```python
from build123d import *

# Parameters (mm, degrees)
ESQUISSE1_R             = 3
BOSS_EXTRU_1_DEPTH      = 10
ESQUISSE2_R             = 2
BOSS_EXTRU_2_DEPTH      = 8
ESQUISSE6_W             = 50
ESQUISSE6_H             = 0.42
BOSS_EXTRU_4_DEPTH      = 10
ESQUISSE7_W             = 50
ESQUISSE7_H             = 0.81
ENL_V_MAT_EXTRU_3_DEPTH = 10
ESQUISSE8_R             = 2
BOSS_EXTRU_5_DEPTH      = 8.39


with BuildPart() as part:
    # Esquisse1 → Boss.-Extru.1 (new body)
    with BuildSketch(Plane.XY):
        with BuildLine():
            Line((-25, -12.35), (25, -12.35))
            Line((25, -12.35), (25, 12.35))
            ThreePointArc((25, 12.35), (0, 37.35), (-25, 12.35))
            Line((-25, 12.35), (-25, -12.35))
        make_face()
        with Locations((0, 12.35)):
            Circle(ESQUISSE1_R, mode=Mode.SUBTRACT)
    extrude(amount=BOSS_EXTRU_1_DEPTH)

    # Esquisse2 → Boss.-Extru.2 (add)
    with BuildSketch(Plane.XZ.offset(12.35)):
        with Locations(Location((-10.94600496, 5, 0), (0, 0, 90))):
            Circle(ESQUISSE2_R)
        with Locations(Location((10.94600496, 5, 0), (0, 0, 90))):
            Circle(ESQUISSE2_R)
    extrude(amount=BOSS_EXTRU_2_DEPTH)

    # Esquisse6 → Boss.-Extru.4 (add)
    with BuildSketch(Plane.XY.offset(10)):
        with Locations((0, -12.56)):
            Rectangle(ESQUISSE6_W, ESQUISSE6_H)
    extrude(amount=-BOSS_EXTRU_4_DEPTH)

    # Esquisse7 → Enl_v. mat.-Extru.3 (cut)
    with BuildSketch(Plane.XY.offset(10)):
        with Locations((0, -12.365)):
            Rectangle(ESQUISSE7_W, ESQUISSE7_H)
    extrude(amount=-ENL_V_MAT_EXTRU_3_DEPTH, mode=Mode.SUBTRACT)


with BuildPart() as enl_v_mat_extru_3_piece_1:
    # of the separate pieces the step leaves, piece 1, a body of its own (enl_v_mat_extru_3_pieces)
    add(part.part.solids().sort_by_distance((-25, 12.35, 0))[0])



with BuildPart() as enl_v_mat_extru_3_piece_2:
    # of the separate pieces the step leaves, piece 2, a body of its own (enl_v_mat_extru_3_pieces)
    add(part.part.solids().sort_by_distance((-10.94600496, -12.77, 7))[0])


with BuildPart() as enl_v_mat_extru_3_piece_3:
    # of the separate pieces the step leaves, piece 3, a body of its own (enl_v_mat_extru_3_pieces)
    add(part.part.solids().sort_by_distance((10.94600496, -12.77, 7))[0])


with BuildPart() as enl_v_mat_extru_3_piece_1_1:
    add(enl_v_mat_extru_3_piece_1.part)

    add(enl_v_mat_extru_3_piece_2.part)  # Boss.-Extru.5 merges Enl_v. mat.-Extru.3 piece 2

    add(enl_v_mat_extru_3_piece_3.part)  # Boss.-Extru.5 merges Enl_v. mat.-Extru.3 piece 3
    # Esquisse8 → Boss.-Extru.5 (add)
    with BuildSketch(Plane.XZ.offset(11.96)):
        with Locations(Location((-10.94600496, 5, 0), (0, 0, 90))):
            Circle(ESQUISSE8_R)
        with Locations(Location((10.94600496, 5, 0), (0, 0, 90))):
            Circle(ESQUISSE8_R)
    extrude(amount=BOSS_EXTRU_5_DEPTH)


solid = enl_v_mat_extru_3_piece_1_1.part
```
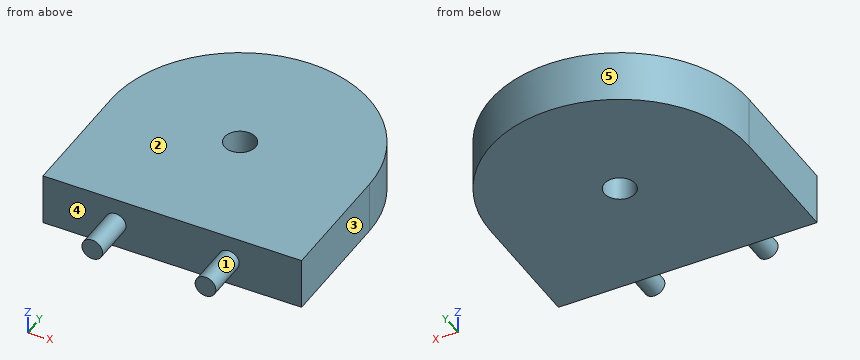
Model file for the job. Use its own axes, mm. Face numbers are marked on the shaded views. A direction names the side the tool comes from. Round coordinates to 2 decimals unless told otherwise and drop trailing zeros. Write each loop counter-clockwise with the first axis right and the second up, starting at its lowest first coordinate (ties: lowest second). Pieces come first, ordered by that corner, then holes. Notation, with made-up numbers: M -22,31 L 10,31 A20 cw 10,61 Z; hole C 48,-10 d6. An arc over 180 degrees is marked long. Put each result on its own line as item: value.
Item 1: Mould opens along X. For the marked faces 3, 4 and 5 say: +X half, -X half, draft (parallel to the pull), parting line (faces both ways), or undercut.
Responses:
face 3: +X half
face 4: undercut
face 5: parting line
Item 2: Cut at A-A (x = 0). List the corners of the cut face in (y, z), and give its area (3 significant figures).
Responses:
outline: M -11.96,0 L 9.35,0 L 9.35,10 L -11.96,10 Z; M 15.35,0 L 37.35,0 L 37.35,10 L 15.35,10 Z
area: 433 mm²
Item 3: Cut at C-C (x = 12). List the corners of the cut face in (y, z).
Responses:
outline: M -20.35,3.3 L -11.96,3.3 L -11.96,0 L 34.28,0 L 34.28,10 L -11.96,10 L -11.96,6.7 L -20.35,6.7 Z
Item 4: Probe L1, parallel to Y at x = 0, z = 3.75; L2, parallel to X at y = 10, z = 8; L3, parallel to X at y = 12, z = 6.25. List the from-to ranges inside material, lowest first. Write a range as from..to.
Responses:
L1: -11.96..9.35, 15.35..37.35
L2: -25..-1.86, 1.86..25
L3: -25..-2.98, 2.98..25
Item 5: Cut at B-B (z = 5). List the corners of the cut face in (x, y), and give its area (3 significant figures).
Responses:
outline: M -25,-11.96 L -12.95,-11.96 L -12.95,-20.35 L -8.95,-20.35 L -8.95,-11.96 L 8.95,-11.96 L 8.95,-20.35 L 12.95,-20.35 L 12.95,-11.96 L 25,-11.96 L 25,12.35 A25 ccw -25,12.35 Z; hole C 0,12.35 d6
area: 2,240 mm²
Item 6: Tool access for the marked faces 1 and 2: list every direction of +Z, -Z, +X, -X, +Y, -Y with a clear straight run to the whole face (end or side of a thin tool).
Responses:
face 1: -Y
face 2: +Z, +X, -X, +Y, -Y
Item 7: Flat gauge pin, fed straight in: P1, Ø6, axis at x = -1, z = 4, coming from the -Y side. Where does the tip first touch, or does it go through?
Responses:
P1: y = -11.96
Item 8: Cut at D-D (z = 1). List the corners of the cut face in (x, y), and give its area (3 significant figures).
Responses:
outline: M -25,-11.96 L 25,-11.96 L 25,12.35 A25 ccw -25,12.35 Z; hole C 0,12.35 d6
area: 2,170 mm²
